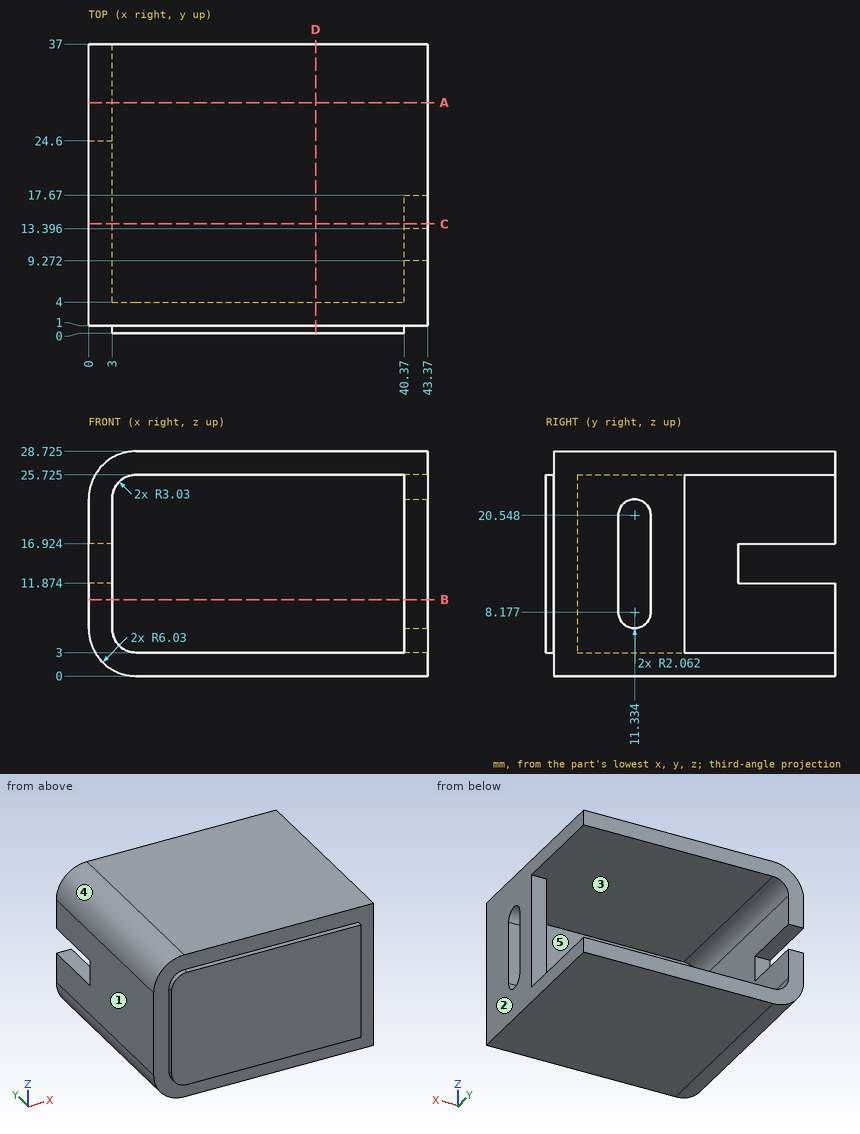
Job drawing, mm, ordinate dimensions from the low corner. One solid piece. A direction names the side the tool comes from. Coordinates: 2 decimals unless noted, no trailing zeros. Order: outer loops, then holes, each group sorted by start corner. A loop starts at its lowest first (then second) coordinate and runs counter-clockwise, first axis right, second up. Notation, with made-up numbers: (71, 11.5) -> (94, 11.5) arc R27 ccw to (94, 28.5) -> close; hole circle Ø5 at (-19, -9). An arc over 180 degrees is marked (long way). Put each result on its own line as item: value. Start each with the question number.
(1) Pin check, flat tips, straight feed: pin 1 Ø1.5 at (x, z) = (2, 14) entering from +Y; pin 2 Ø1.5 at (x, z) = (42, 17) entering from -Y; pin 3 Ø0.5 at (y, z) = (0.5, 11.5) entering from -X. Stop position of each tip, or through.
(2) Which spindle directions (+Z, -Z, +X, -X, +Y, -Y) get a long thin tool onto all of the face, cutting with end or side? Do the marked faces 4 and 5. Say none if no direction does.
(3) Band-saw the part on B-B (z = 9.75). Give the cut face in (x, y) (1 decimal), then the cut area to 3 significant figures.
(4) Band-saw the part on D-D (x = 29). Give the cut face in (y, z) (1 decimal), then the cut area to 3 significant figures.
(5) Probe line 1 along Z through (x, y) = (39, 25) (1 decimal); line 2 along Y through (x, z) = (40.5, 9) (1 decimal); line 3 along X through (y, z) = (25, 21). List the from-to ranges inside material, lowest first. Write a range as [from, to].
(6) Band-saw the part on A-A (y = 29.5). Give the cut face in (x, z) (1 decimal).
(7) Mould opens along X. For the marked faces 1, 2 and 3 say: pulls with the +X half, pulls with the -X half, needs draft (parallel to the pull), parting line crosses it, or undercut.
(8) Band-saw the part on C-C (y = 14). Give the cut face in (x, z) (1 decimal), then the cut area to 3 significant figures.
Determined:
1. pin 1: stops at y = 24.6
1. pin 2: stops at y = 1
1. pin 3: stops at x = 3
2. face 4: +Z, -X, +Y, -Y
2. face 5: +Y
3. outline: (0, 1) -> (3, 1) -> (3, 0) -> (40.4, 0) -> (40.4, 1) -> (43.4, 1) -> (43.4, 9.3) -> (40.4, 9.3) -> (40.4, 4) -> (3, 4) -> (3, 37) -> (0, 37) -> close; (40.4, 13.4) -> (43.4, 13.4) -> (43.4, 17.7) -> (40.4, 17.7) -> close
3. area: 295 mm²
4. outline: (0, 3) -> (1, 3) -> (1, 0) -> (37, 0) -> (37, 3) -> (4, 3) -> (4, 25.7) -> (37, 25.7) -> (37, 28.7) -> (1, 28.7) -> (1, 25.7) -> (0, 25.7) -> close
4. area: 307 mm²
5. line 1: z = [0, 3], [25.7, 28.7]
5. line 2: y = [1, 9.3], [13.4, 17.7]
5. line 3: x = [0, 3]
6. outline: (0, 6) arc R6 ccw to (6, 0) -> (43.4, 0) -> (43.4, 3) -> (6, 3) arc R3 cw to (3, 6) -> (3, 11.9) -> (0, 11.9) -> close; (0, 16.9) -> (3, 16.9) -> (3, 22.7) arc R3 cw to (6, 25.7) -> (43.4, 25.7) -> (43.4, 28.7) -> (6, 28.7) arc R6 ccw to (0, 22.7) -> close
7. face 1: pulls with the -X half
7. face 2: pulls with the +X half
7. face 3: undercut
8. outline: (0, 6) arc R6 ccw to (6, 0) -> (43.4, 0) -> (43.4, 28.7) -> (6, 28.7) arc R6 ccw to (0, 22.7) -> close; hole (3, 6) arc R3 ccw to (6, 3) -> (40.4, 3) -> (40.4, 25.7) -> (6, 25.7) arc R3 ccw to (3, 22.7) -> close
8. area: 385 mm²
